```python
from build123d import *

# Parameters (mm, degrees)
SKETCH1_W           = 30
SKETCH1_H           = 8
BOSS_EXTRUDE1_DEPTH = 70
CUT_EXTRUDE1_DEPTH  = 70
SKETCH5_R           = 1.4
CUT_EXTRUDE3_DEPTH  = 100


with BuildPart() as part:
    # Sketch1 → Boss-Extrude1 (new body)
    with BuildSketch(Plane.XY):
        Rectangle(SKETCH1_W, SKETCH1_H)
    extrude(amount=BOSS_EXTRUDE1_DEPTH)

    # Sketch4 → Cut-Extrude1 (cut)
    with BuildSketch(Plane(origin=(0, 4, 0), x_dir=(1, 0, 0), z_dir=(0, 1, 0))):
        Polygon((-15, 0), (-10, 0), (-15, -70), align=None)
        Polygon((15, 0), (10, 0), (15, -70), align=None)
    extrude(amount=-CUT_EXTRUDE1_DEPTH, mode=Mode.SUBTRACT)

    # Sketch5 → Cut-Extrude3 (cut)
    with BuildSketch(Plane(origin=(0, 4, 0), x_dir=(1, 0, 0), z_dir=(0, 1, 0))):
        with Locations(Location((0, -3.6, 0), (0, 0, 180))):
            Circle(SKETCH5_R)
    extrude(amount=-CUT_EXTRUDE3_DEPTH, mode=Mode.SUBTRACT)


solid = part.part
```
Geometry check sheet. Reference: the model listing, model coordinates, mm. Round coordinates to 2 decimals unless told otherwise and drop trailing zeros. Loops run counter-clockwise (first coordinate to the right, second up) from the corner with the lowest first, then second, coordinate; pieces in that order, holes last. Notation, with made-up numbers: M 59.5,86 L 85.5,86 A29 cw 85.5,112 Z; hole C 71,-27.5 d11. An arc over 180 degrees is marked long. Return JSON: item names as keys, results as strings. Group by question number.
(1) Go/stop test with flat-tipped pins: pin 1 (2 mm diameter, centred on x = 0, z = 3.6, fed in from +Y); pin 2 (1.5 mm diameter, centred on y = -1, z = 50.5, fed in from -X); pin 3 (1 mm diameter, centred on y = -1, z = 59, fed in from +X). Record where each tip stops, or that it passes through.
(2) Section check D-D, the plane z = 28.5. Enter the section's corners in (x, y), and give its area (3 significant figures).
(3) Section check A-A, the plane x = 0. Enter the section's corners in (y, z), and give its area (3 significant figures).
(4) Mould release check, pull along X, two halves, no side actions. Record for faces 1 (the face through (-0.75, 0.06, 4.78)), 2 (the face through (12.465, 0.056, 34.51)), 3 (the face through (-12.465, 0.056, 34.51)), 4 (the face through (0, -4, 35)): pulls with the +X half, pulls with the -X half, needs draft (parallel to the pull), parting line crosses it, or undercut.
(5) Scan lines: line 1 along Z through (x, y) = (0, 0.5); line 2 along X through (y, z) = (-0.75, 62); line 3 along X through (y, z) = (1.25, 6). Record each from-to range of solid material in increasing order. Write a range as [from, to].
(6) Section check C-C, the plane z = 3.6. Enter the section's corners in (x, y), and give its area (3 significant figures).
(7) Section check B-B, the plane y = -0.75. Enter the section's corners in (x, z), and give its area (3 significant figures).
Data:
{
 "1": {"pin 1": "through", "pin 2": "x = -13.66", "pin 3": "x = 14.25"},
 "2": {"outline": "M -12.04,-4 L 12.04,-4 L 12.04,4 L -12.04,4 Z", "area": "193 mm²"},
 "3": {"outline": "M -4,0 L 4,0 L 4,2.2 L -4,2.2 Z; M -4,5 L 4,5 L 4,70 L -4,70 Z", "area": "538 mm²"},
 "4": {"face 1": "undercut", "face 2": "pulls with the +X half", "face 3": "pulls with the -X half", "face 4": "needs draft"},
 "5": {"line 1": "[0, 2.2], [5, 70]", "line 2": "[-14.43, 14.43]", "line 3": "[-10.43, 10.43]"},
 "6": {"outline": "M -10.26,-4 L -1.4,-4 L -1.4,4 L -10.26,4 Z; M 1.4,-4 L 10.26,-4 L 10.26,4 L 1.4,4 Z", "area": "142 mm²"},
 "7": {"outline": "M -15,70 L -10,0 L 10,0 L 15,70 Z; hole C 0,3.6 d2.8", "area": "1,740 mm²"}
}
